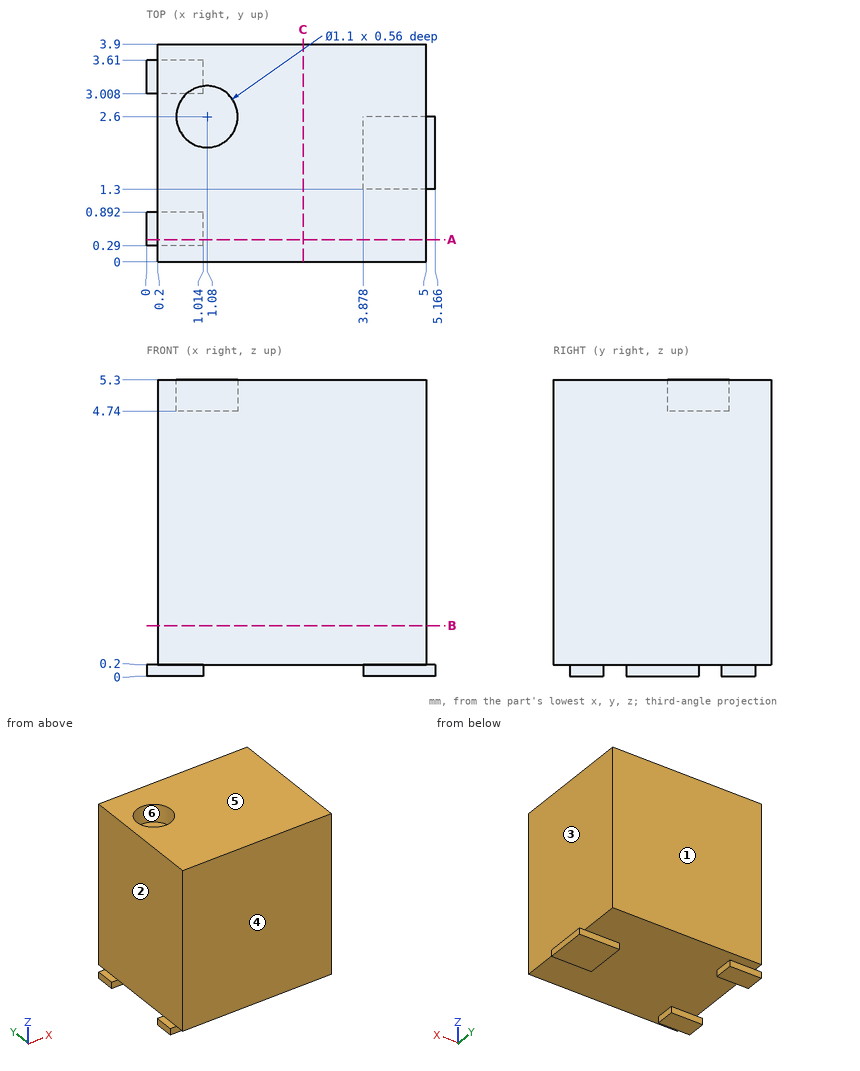
Part print with two shaded views. Sizes in mm from the minimum x, y, z corner. A direction names the side the tool comes from. Coordinates: 2 decimals unless noted, no trailing zeros. Loops run counter-clockwise (first coordinate to the right, second up) from the corner with the lowest first, then second, coordinate; pieces in that order, holes last. Notation, with made-up numbers: (-39, 61.25) -> (-19, 61.25) arc R32 ccw to (-19, 93.25) -> close; hole circle Ø2 at (64.5, -1.75). An arc over 180 degrees is marked (long way). Answer as a JSON object with one key per item and string values.
Q1. 3-axis set-ups, long thin cutter, end or side, ignore diameter. For the marked faces 1, 2 and 3: which of +Z, -Z, +X, -X, +Y, -Y reach the whole face in a straight line?
Report:
{"face 1": "+Z, -Z, +X, -X, +Y", "face 2": "+Z, -X, +Y, -Y", "face 3": "+Z, +X, +Y, -Y"}
Q2. Cut at A-A (y = 0.4). List the corners of the cut face in (x, z).
Report:
{"outline": "(0, 0) -> (1.01, 0) -> (1.01, 0.2) -> (5, 0.2) -> (5, 5.3) -> (0.2, 5.3) -> (0.2, 0.2) -> (0, 0.2) -> close"}
Q3. Cut at C-C (x = 2.8). List the corners of the cut face in (y, z).
Report:
{"outline": "(0, 0.2) -> (3.9, 0.2) -> (3.9, 5.3) -> (0, 5.3) -> close"}
Q4. Cut at B-B (z = 0.9). List the corners of the cut face in (x, y), and give its area (3 significant figures).
Report:
{"outline": "(0.2, 0) -> (5, 0) -> (5, 3.9) -> (0.2, 3.9) -> close", "area": "18.7 mm2"}
Q5. Flat gauge pins, fed straight in: P1, Ø1.5, axis at y = 2, z = 4, coming from the -X side; P2, Ø1.5, axis at x = 3, y = 2.5, coming from the -Z side. Where does each tip first touch, or does it go through?
Report:
{"P1": "stops at x = 0.2", "P2": "stops at z = 0.2"}
Q6. Probe probe 1 along Y at (x, z) = (1.08, 4.9); probe 2 along X at (y, z) = (3.65, 4.75); probe 3 along Z at (x, y) = (3.4, 1). List the from-to ranges inside material, lowest first.
Report:
{"probe 1": "y = 0 to 2.05, 3.15 to 3.9", "probe 2": "x = 0.2 to 5", "probe 3": "z = 0.2 to 5.3"}
Q7. Pull direction Y, two halves, no side cores. Call the marked faces 4, 5 and 6: released by +Y, released by -Y, zero draft, split by the parting line, or undercut.
Report:
{"face 4": "released by -Y", "face 5": "zero draft", "face 6": "undercut"}
